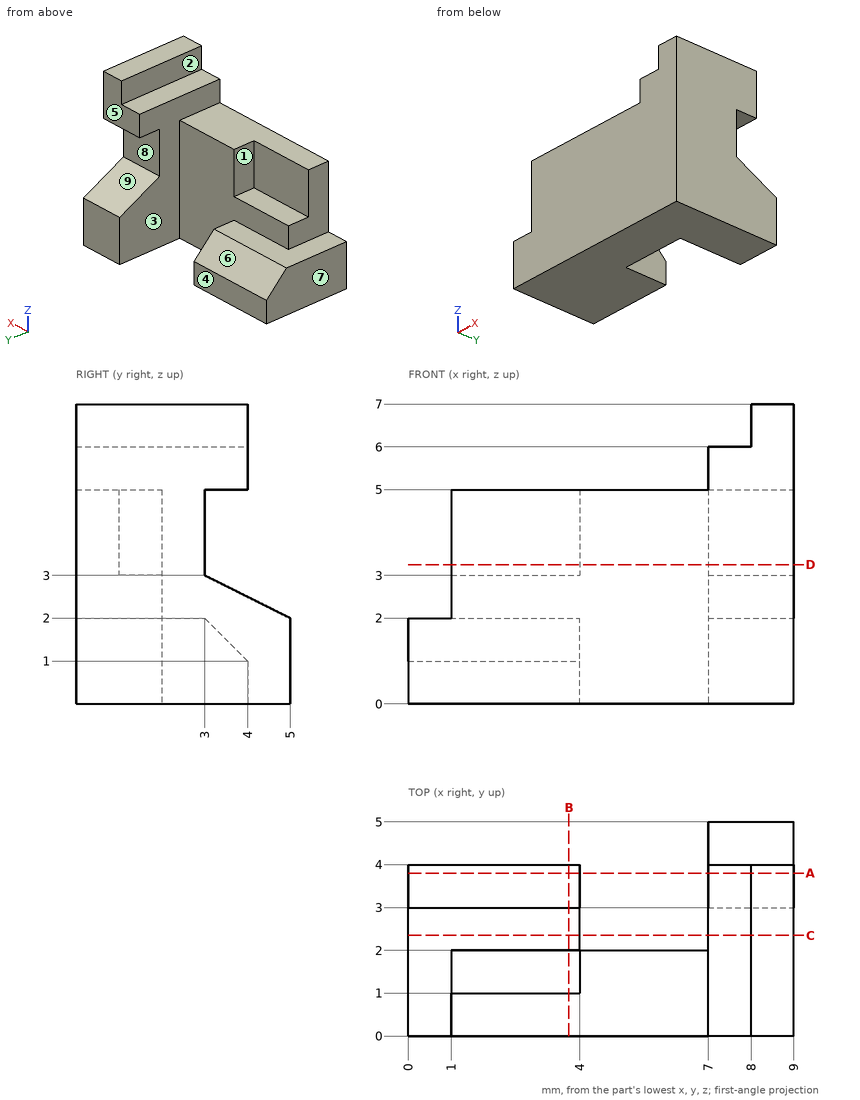
Drawing for the job (mm, zero at the part's lowest x, y, z). A direction names the side the tool comes from. Round coordinates to 2 decimals unless told otherwise and drop trailing zeros. Write each loop counter-clockwise with the first axis right and the second up, starting at its lowest first coordinate (ties: lowest second). Pieces come first, ordered by that corner, then holes. Notation, with made-up numbers: (26.25, 9) - (77.25, 9) arc R11 ccw to (77.25, 28) - close; hole circle Ø1 at (56, 37.25). An arc over 180 degrees is marked (long way). Write item = value, one per line. Start each with the question number.
Q1. Which spindle directions (+Z, -Z, +X, -X, +Y, -Y) get a long thin tool onto all of the face, cutting with end or side? Do the marked faces 1, 2, 3, 4 and 5. Say none if no direction does.
Q2. Band-saw the part on C-C (y = 2.35). Give the cut face in (x, z), then the cut area to 3 significant figures.
Q3. Band-saw the part on A-A (y = 3.8). Give the cut face in (x, z).
Q4. Drop flat-ended pins along their axis: pin 1 (2 mm diameter, centred on x = 8, z = 3.5, fed in from +Y); pin 2 (1.5 mm diameter, centred on x = 2, y = 1.5, fed in from +Z); pin 3 (1.6 mm diameter, centred on y = 1, z = 3.5, fed in from -X). Give the stop position or say it passes through.
Q5. Mould opens along Z. For the marked faces 6, 7, 8 and 9 say: pulls with the +Z half, pulls with the -Z half, needs draft (parallel to the pull), parting line crosses it, or undercut.
Q6. Probe L1, parallel to X at y = 2.8, z = 1.75; L2, parallel to X at y = 2.55, z = 3; L3, parallel to Z at x = 2, y = 0.4. List the from-to ranges inside material, lowest first. Write a range as from..to.
Q7. Band-saw the part on D-D (z = 3.25). Give the cut face in (x, y).
Q8. Band-saw the part on B-B (x = 3.75). Give the cut face in (y, z).
Answers below:
q1.face_1 = +Z, -X, +Y
q1.face_2 = +Z, -X, +Y, -Y
q1.face_3 = +Z, +Y
q1.face_4 = +Z, -Z, -X, +Y
q1.face_5 = +Z, +X, -X, +Y
q2.outline = (0, 0) - (4, 0) - (4, 2) - (0, 2) - close; (7, 0) - (9, 0) - (9, 7) - (8, 7) - (8, 6) - (7, 6) - close
q2.area = 21.0 mm2
q3.outline = (0, 0) - (4, 0) - (4, 1.2) - (0, 1.2) - close; (7, 0) - (9, 0) - (9, 2.6) - (7, 2.6) - close; (7, 5) - (9, 5) - (9, 7) - (8, 7) - (8, 6) - (7, 6) - close
q4.pin_1 = 4
q4.pin_2 = 5
q4.pin_3 = 1
q5.face_6 = pulls with the +Z half
q5.face_7 = needs draft
q5.face_8 = undercut
q5.face_9 = undercut
q6.L1 = 0..4, 7..9
q6.L2 = 7..9
q6.L3 = 0..5
q7.outline = (1, 0) - (9, 0) - (9, 3) - (7, 3) - (7, 2) - (4, 2) - (4, 1) - (1, 1) - close
q8.outline = (0, 0) - (4, 0) - (4, 1) - (3, 2) - (2, 2) - (2, 3) - (1, 3) - (1, 5) - (0, 5) - close
